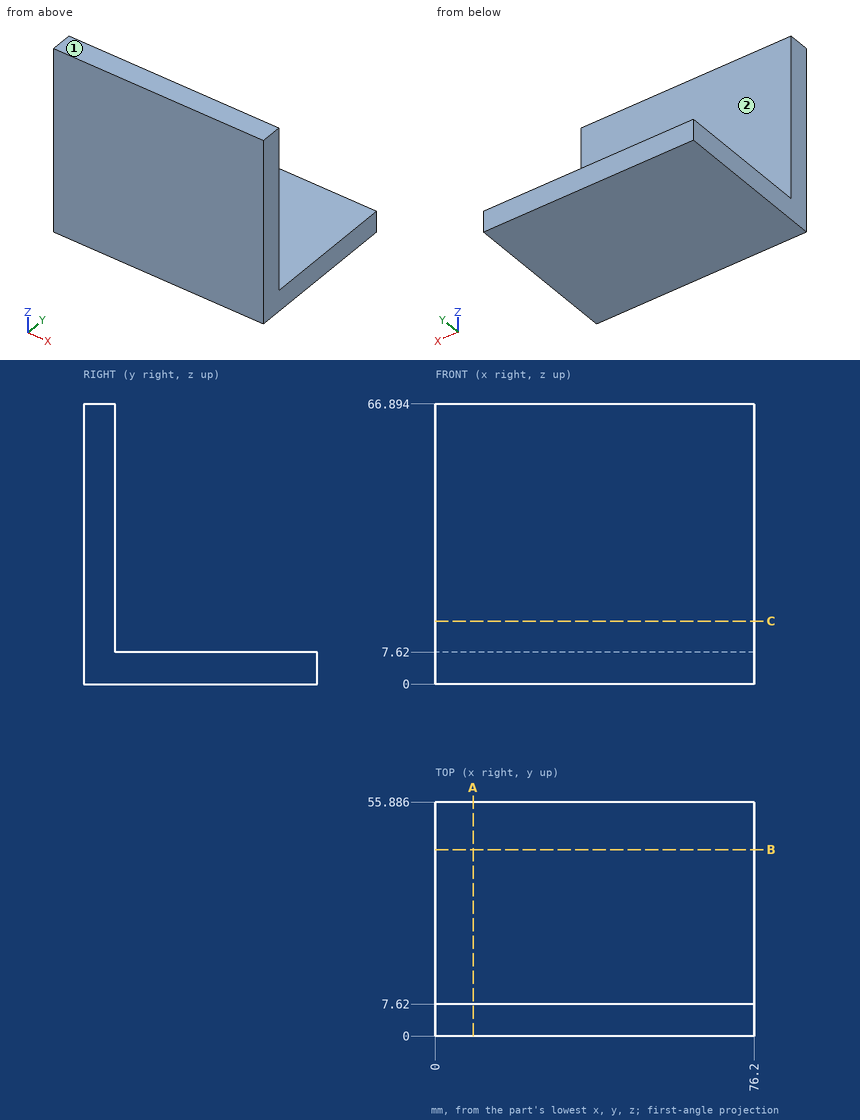
Study the drawing (mm; zero at the part's minimum x, y, z) and answer. A direction names the side the tool comes from. Give positions to 0.01 mm unless a question says otherwise; leave off trailing zeros. Loops run counter-clockwise (first coordinate to the right, second up) from the corner with the lowest first, then second, coordinate; pieces in that order, holes last. Notation, with made-up numbers: M 34.5,15 L 58.5,15 A23 cw 58.5,33 Z; hole C 8,64 d1. An arc over 180 degrees is marked long. Answer as CSV lines item,"result".
Item 1: A straight line is drawn through the part: line 1 along Z through (x, y) = (22.5, 23). Find the intervals that lie inside material, in ascending order. Write a range as [from, to].
Values follow:
line 1,"z = [0, 7.62]"
Item 2: The part is cut by section B-B (y = 44.5). Give the vertices of the cut face in (x, z).
Values follow:
outline,"M 0,0 L 76.2,0 L 76.2,7.62 L 0,7.62 Z"
Item 3: Which of the six approach directions +Z, -Z, +X, -X, +Y, -Y give full straight-line access (tool end or side, diameter ignored) to the marked faces 1 and 2?
Values follow:
face 1,"+Z, +X, -X, +Y, -Y"
face 2,"+Z, +X, -X, +Y"
Item 4: Given pin 1 Ø14.5 at (x, y) = (38, 23.5) entering from +Z; pin 2 Ø2 at (x, y) = (24, 11.5) entering from -Z; pin 3 Ø4 at (x, z) = (54, 15) entering from +Y, each flat-ended and moving along its own axis, determine where each tip first touches the part or whether it passes through.
Values follow:
pin 1,"stops at z = 7.62"
pin 2,"stops at z = 0"
pin 3,"stops at y = 7.62"
Item 5: The part is cut by section A-A (x = 9). Give the vertices of the cut face in (y, z).
Values follow:
outline,"M 0,0 L 55.89,0 L 55.89,7.62 L 7.62,7.62 L 7.62,66.89 L 0,66.89 Z"
